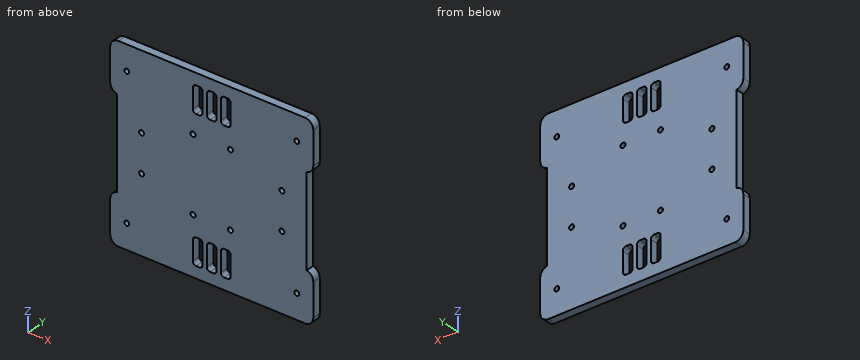
from build123d import *

# Parameters (mm, degrees)
RESSALTO_EXTRUS_O1_DEPTH = 5
FILETE1_R                = 5
ESBO_O3_R                = 1.5
CORTE_EXTRUS_O1_DEPTH    = 5
ESBO_O5_R                = 1.5
CORTE_EXTRUS_O2_DEPTH    = 10


with BuildPart() as part:
    # Esboço1 → Ressalto-extrusão1 (new body)
    with BuildSketch(Plane(origin=(0, 0, 0), x_dir=(1, 0, 0), z_dir=(0, 1, 0))):
        with BuildLine():
            Line((81.90590785, -20.429188404), (85.90590785, -20.429188404))
            Line((85.90590785, -20.429188404), (85.90590785, 4.570811596))
            ThreePointArc((85.90590785, 4.570811596), (84.441441756, 8.106345502), (80.90590785, 9.570811596))
            Line((80.90590785, 9.570811596), (-32.09409215, 9.570811596))
            ThreePointArc((-32.09409215, 9.570811596), (-35.629626056, 8.106345502), (-37.09409215, 4.570811596))
            Line((-37.09409215, 4.570811596), (-37.09409215, -20.429188404))
            Line((-37.09409215, -20.429188404), (-33.09409215, -20.429188404))
            Line((-33.09409215, -20.429188404), (-33.09409215, -75.429188404))
            Line((-33.09409215, -75.429188404), (-37.09409215, -75.429188404))
            Line((-37.09409215, -75.429188404), (-37.09409215, -100.429188404))
            ThreePointArc((-37.09409215, -100.429188404), (-35.629626056, -103.96472231), (-32.09409215, -105.429188404))
            Line((-32.09409215, -105.429188404), (80.90590785, -105.429188404))
            ThreePointArc((80.90590785, -105.429188404), (84.441441756, -103.96472231), (85.90590785, -100.429188404))
            Line((85.90590785, -100.429188404), (85.90590785, -75.429188404))
            Line((85.90590785, -75.429188404), (81.90590785, -75.429188404))
            Line((81.90590785, -75.429188404), (81.90590785, -20.429188404))
        make_face()
    extrude(amount=RESSALTO_EXTRUS_O1_DEPTH)

    # Filete1
    # the kernel refuses this fillet: 5 mm, written as the material it takes off along each edge
    with BuildSketch(Plane(origin=(-37.09409215, -12.247448714, 75.429188404), x_dir=(1.0, 0, 1.5738521597081158e-12), z_dir=(0, 1, 0)), Plane(origin=(85.90590785, -12.247448714, 20.429188404), x_dir=(-1.0, 0, -1.5685230891899197e-12), z_dir=(0, 1, 0))) as filete1_piece_1:
        with BuildLine():
            CenterArc((5, -4.898979486), FILETE1_R, 101.536959033, 78.463040967)
            Line((0, -4.898979486), (-0.1, -4.898979486))
            Line((-0.1, -4.898979486), (-0.1, 0))
            Line((-0.1, 0), (0, 0.1))
            ThreePointArc((0, 0.1), (2, 0.1), (3.98, 0.09797959))
            Line((3.98, 0.09797959), (4, 0))
        make_face()
    extrude(amount=29.494897428, mode=Mode.SUBTRACT)
    with BuildSketch(Plane(origin=(-37.09409215, -12.247448714, 20.429188404), x_dir=(0, 0, -1), z_dir=(0, 1, 0)), Plane(origin=(85.90590785, -12.247448714, 75.429188404), x_dir=(0, 0, 1), z_dir=(0, 1, 0))) as filete1_piece_2:
        with BuildLine():
            CenterArc((4.898979486, -5), FILETE1_R, 90, 78.463040967)
            Line((0, -4), (-0.09797959, -3.98))
            ThreePointArc((-0.09797959, -3.98), (-0.1, -2), (-0.1, 0))
            Line((-0.1, 0), (0, 0.1))
            Line((0, 0.1), (4.898979486, 0.1))
            Line((4.898979486, 0.1), (4.898979486, 0))
        make_face()
    extrude(amount=29.494897428, mode=Mode.SUBTRACT)

    # Esboço3 → Corte-extrusão1 (cut)
    with BuildSketch(Plane.XZ):
        with Locations(Location((-27.09409215, 5.429188404, 0), (0, 0, 270))):
            Circle(ESBO_O3_R)
        with Locations(Location((75.90590785, 5.429188404, 0), (0, 0, 270))):
            Circle(ESBO_O3_R)
        with Locations(Location((75.90590785, 90.429188404, 0), (0, 0, 90))):
            Circle(ESBO_O3_R)
        with Locations(Location((-27.09409215, 90.429188404, 0), (0, 0, 90))):
            Circle(ESBO_O3_R)
        with BuildLine():
            Line((35.90590785, 84.429188404), (35.90590785, 96.429188404))
            ThreePointArc((35.90590785, 96.429188404), (35.320121412, 97.843401966), (33.90590785, 98.429188404))
            Line((33.90590785, 98.429188404), (31.90590785, 98.429188404))
            ThreePointArc((31.90590785, 98.429188404), (30.491694287, 97.843401966), (29.90590785, 96.429188404))
            Line((29.90590785, 96.429188404), (29.90590785, 84.429188404))
            ThreePointArc((29.90590785, 84.429188404), (30.491694287, 83.014974841), (31.90590785, 82.429188404))
            Line((31.90590785, 82.429188404), (33.90590785, 82.429188404))
            ThreePointArc((33.90590785, 82.429188404), (35.320121412, 83.014974841), (35.90590785, 84.429188404))
        make_face()
        with BuildLine():
            Line((14.90590785, 13.429188404), (16.90590785, 13.429188404))
            ThreePointArc((16.90590785, 13.429188404), (18.320121412, 12.843401966), (18.90590785, 11.429188404))
            Line((18.90590785, 11.429188404), (18.90590785, -0.570811596))
            ThreePointArc((18.90590785, -0.570811596), (18.320121412, -1.985025159), (16.90590785, -2.570811596))
            Line((16.90590785, -2.570811596), (14.90590785, -2.570811596))
            ThreePointArc((14.90590785, -2.570811596), (13.491694287, -1.985025159), (12.90590785, -0.570811596))
            Line((12.90590785, -0.570811596), (12.90590785, 11.429188404))
            ThreePointArc((12.90590785, 11.429188404), (13.491694287, 12.843401966), (14.90590785, 13.429188404))
        make_face()
        with BuildLine():
            Line((23.40590785, 13.429188404), (25.40590785, 13.429188404))
            ThreePointArc((25.40590785, 13.429188404), (26.820121412, 12.843401966), (27.40590785, 11.429188404))
            Line((27.40590785, 11.429188404), (27.40590785, -0.570811596))
            ThreePointArc((27.40590785, -0.570811596), (26.820121412, -1.985025159), (25.40590785, -2.570811596))
            Line((25.40590785, -2.570811596), (23.40590785, -2.570811596))
            ThreePointArc((23.40590785, -2.570811596), (21.991694287, -1.985025159), (21.40590785, -0.570811596))
            Line((21.40590785, -0.570811596), (21.40590785, 11.429188404))
            ThreePointArc((21.40590785, 11.429188404), (21.991694287, 12.843401966), (23.40590785, 13.429188404))
        make_face()
        with BuildLine():
            Line((31.90590785, 13.429188404), (33.90590785, 13.429188404))
            ThreePointArc((33.90590785, 13.429188404), (35.320121412, 12.843401966), (35.90590785, 11.429188404))
            Line((35.90590785, 11.429188404), (35.90590785, -0.570811596))
            ThreePointArc((35.90590785, -0.570811596), (35.320121412, -1.985025159), (33.90590785, -2.570811596))
            Line((33.90590785, -2.570811596), (31.90590785, -2.570811596))
            ThreePointArc((31.90590785, -2.570811596), (30.491694287, -1.985025159), (29.90590785, -0.570811596))
            Line((29.90590785, -0.570811596), (29.90590785, 11.429188404))
            ThreePointArc((29.90590785, 11.429188404), (30.491694287, 12.843401966), (31.90590785, 13.429188404))
        make_face()
        with BuildLine():
            Line((27.40590785, 84.429188404), (27.40590785, 96.429188404))
            ThreePointArc((27.40590785, 96.429188404), (26.820121412, 97.843401966), (25.40590785, 98.429188404))
            Line((25.40590785, 98.429188404), (23.40590785, 98.429188404))
            ThreePointArc((23.40590785, 98.429188404), (21.991694287, 97.843401966), (21.40590785, 96.429188404))
            Line((21.40590785, 96.429188404), (21.40590785, 84.429188404))
            ThreePointArc((21.40590785, 84.429188404), (21.991694287, 83.014974841), (23.40590785, 82.429188404))
            Line((23.40590785, 82.429188404), (25.40590785, 82.429188404))
            ThreePointArc((25.40590785, 82.429188404), (26.820121412, 83.014974841), (27.40590785, 84.429188404))
        make_face()
        with BuildLine():
            Line((18.90590785, 84.429188404), (18.90590785, 96.429188404))
            ThreePointArc((18.90590785, 96.429188404), (18.320121412, 97.843401966), (16.90590785, 98.429188404))
            Line((16.90590785, 98.429188404), (14.90590785, 98.429188404))
            ThreePointArc((14.90590785, 98.429188404), (13.491694287, 97.843401966), (12.90590785, 96.429188404))
            Line((12.90590785, 96.429188404), (12.90590785, 84.429188404))
            ThreePointArc((12.90590785, 84.429188404), (13.491694287, 83.014974841), (14.90590785, 82.429188404))
            Line((14.90590785, 82.429188404), (16.90590785, 82.429188404))
            ThreePointArc((16.90590785, 82.429188404), (18.320121412, 83.014974841), (18.90590785, 84.429188404))
        make_face()
    extrude(amount=-CORTE_EXTRUS_O1_DEPTH, mode=Mode.SUBTRACT)

    # Esboço5 → Corte-extrusão2 (cut)
    with BuildSketch(Plane.XZ):
        with Locations(Location((13.05590785, 25.429188404, 0), (0, 0, 270))):
            Circle(ESBO_O5_R)
        with Locations(Location((35.75590785, 25.429188404, 0), (0, 0, 270))):
            Circle(ESBO_O5_R)
        with Locations(Location((-18.09409215, 59.279188404, 0), (0, 0, 270))):
            Circle(ESBO_O5_R)
        with Locations(Location((-18.09409215, 36.579188404, 0), (0, 0, 270))):
            Circle(ESBO_O5_R)
        with Locations(Location((13.05590785, 70.429188404, 0), (0, 0, 90))):
            Circle(ESBO_O5_R)
        with Locations(Location((35.75590785, 70.429188404, 0), (0, 0, 90))):
            Circle(ESBO_O5_R)
        with Locations(Location((66.90590785, 36.579188404, 0), (0, 0, 90))):
            Circle(ESBO_O5_R)
        with Locations(Location((66.90590785, 59.279188404, 0), (0, 0, 90))):
            Circle(ESBO_O5_R)
    extrude(amount=-CORTE_EXTRUS_O2_DEPTH, mode=Mode.SUBTRACT)


solid = part.part
Read the model definition and answer for the solid it produces. Units are mm, in the model's axes. Round coordinates to 2 decimals unless told otherwise and drop trailing zeros. Order: outer loops, then holes, each group sorted by start corner. A loop starts at its lowest first (then second) coordinate and runs counter-clockwise, first axis right, second up.
1) Flat-ended cylindrical pins translate along their axes: pin 1 (2.5 mm diameter, centred on x = 75.91, z = 5.43, fed in from -Y); pin 2 (3 mm diameter, centred on y = 1.5, z = 57, fed in from -X); pin 3 (1 mm diameter, centred on y = 3, z = 46.5, fed in from +X). Find the tip coordinate at first contact, or state that the pin passes through.
2) Straight lines are drawn through the part: L1, parallel to X at y = 2.25, z = 2.5; L2, parallel to Z at x = 36, y = 3.85; L3, parallel to Z at x = 66, y = 3.7. For each, find the intervals that lie inside material, in ascending order.
3) The part is cut by section A-A on z = 86. Write down the section's boundary in (x, y), plus the area to 3 significant figures.
4) The part is cut by section B-B on z = 42. Write down the section's boundary in (x, y).
5) The part is cut by section C-C on y = 1.15. Give the number of separate pieces and of enclosed holes in the cut face, plus the area to 3 significant figures.
Resolved:
1. pin 1: passes through
1. pin 2: stops at x = -33.09
1. pin 3: stops at x = 81.91
2. L1: x = -37.09 to 12.91, 18.91 to 21.41, 27.41 to 29.91, 35.91 to 85.91
2. L2: z = -9.57 to 23.95, 26.91 to 68.95, 71.91 to 105.43
2. L3: z = -9.57 to 35.38, 37.77 to 58.08, 60.47 to 105.43
3. outline: (-37.09, 0) - (12.91, 0) - (12.91, 5) - (-37.09, 5) - close; (18.91, 0) - (21.41, 0) - (21.41, 5) - (18.91, 5) - close; (27.41, 0) - (29.91, 0) - (29.91, 5) - (27.41, 5) - close; (35.91, 0) - (85.91, 0) - (85.91, 5) - (35.91, 5) - close
3. area: 525 mm2
4. outline: (-33.09, 0) - (81.91, 0) - (81.91, 5) - (-33.09, 5) - close
5. separate pieces: 1
5. enclosed holes: 18
5. area: 13,000 mm2
